from build123d import *

# Parameters (mm, degrees)
ESBO_O1_R                = 1
RESSALTO_EXTRUS_O1_DEPTH = 2.6
ESBO_O2_W                = 9.5
ESBO_O2_H                = 2.6
RESSALTO_EXTRUS_O2_DEPTH = 6
RESSALTO_EXTRUS_O2_TAPER = -20
RESSALTO_EXTRUS_O3_DEPTH = 5


with BuildPart() as part:
    # Esboço1 → Ressalto-extrusão1 (new body)
    with BuildSketch(Plane.XY):
        Polygon((-2.5, 31), (2.5, 31), (2.5, 19), (4.75, 19), (4.75, 0), (-4.75, 0), (-4.75, 19), (-2.5, 19), align=None)
        with Locations((0, 14)):
            Circle(ESBO_O1_R, mode=Mode.SUBTRACT)
    extrude(amount=RESSALTO_EXTRUS_O1_DEPTH)

    # Esboço2 → Ressalto-extrusão2 (add)
    with BuildSketch(Plane.XZ):
        with Locations((0, 1.3)):
            Rectangle(ESBO_O2_W, ESBO_O2_H)
    extrude(amount=-RESSALTO_EXTRUS_O2_DEPTH, taper=RESSALTO_EXTRUS_O2_TAPER)

    # Esboço3 → Ressalto-extrusão3 (add)
    with BuildSketch(Plane(origin=(2.5, 0, 0), x_dir=(0, 0, -1), z_dir=(1, 0, 0))):
        Polygon((-2.6, 31), (-3.6, 31), (-2.6, 25), align=None)
    extrude(amount=-RESSALTO_EXTRUS_O3_DEPTH)


solid = part.part
Geometry check sheet. Reference: the model listing, model coordinates, mm. A direction names the side the tool comes from. Give positions to 0.01 mm unless a question says otherwise; leave off trailing zeros. Order: outer loops, then holes, each group sorted by start corner. A loop starts at its lowest first (then second) coordinate and runs counter-clockwise, first axis right, second up. Notation, with made-up numbers: M -14.5,48 L 0.5,48 A26 ccw 0.5,73 Z; hole C 15,-23 d9. An arc over 180 degrees is marked long. Use a Markdown table: item, result.
Item 1: Depth check by flat-ended pin: P1, Ø7.5, axis at x = 2.5, y = 21, coming from the -Z side; P2, Ø1.6, axis at x = 0, y = 14, coming from the +Z side; P3, Ø3, axis at y = 14.5, z = 2, coming from the +X side; P4, Ø1.1, axis at y = 27.5, z = 2, coming from the +X side. Enter the tip coordinate at first touch or a pass-through.
Answers follow:
| item | result |
|---|---|
| P1 | stops at z = 0 |
| P2 | passes through |
| P3 | stops at x = 4.75 |
| P4 | stops at x = 2.5 |
Item 2: Section check A-A (y = 14). Record the cut outline in (x, z), and give its area (3 significant figures).
Answers follow:
| item | result |
|---|---|
| outline | M -4.75,0 L -1,0 L -1,2.6 L -4.75,2.6 Z; M 1,0 L 4.75,0 L 4.75,2.6 L 1,2.6 Z |
| area | 19.5 mm2 |
Item 3: Draft check along X on faces 1 (the cylindrical face through (0, 13, 1)), 2 (the flat face through (-4.75, 12, 1)), 3 (the flat face through (-4, 19, 1)). Enter one of: +X half, -X half, draft (parallel to the pull), parting line (faces both ways), or undercut.
Answers follow:
| item | result |
|---|---|
| face 1 | undercut |
| face 2 | -X half |
| face 3 | draft |
Item 4: Tool access check on faces 4 (the flat face through (0, 16, 0)), 5 (the flat face through (-2.5, 25, 1)), 6 (the flat face through (0, 31, 2)), 7 (the flat face through (0, 28, 3.1)), 8 (the flat face through (4.75, 13, 1)). Record the directions out of +Z, -Z, +X, -X, +Y, -Y that give a thin tool (end or side, any length) a straight path to the whole face; none if there is none.
Answers follow:
| item | result |
|---|---|
| face 4 | -Z, +X, -X, +Y |
| face 5 | +Z, -Z, -X, +Y |
| face 6 | +Z, -Z, +X, -X, +Y |
| face 7 | +Z, +X, -X |
| face 8 | +Z, -Z, +X, +Y |
Item 5: Material ranges on line 1 along Y through (x, z) = (0, 1.9); line 2 along Y through (x, z) = (-2.75, 1.5); line 3 along Z through (x, y) = (4, 15), recorded low to high.
Answers follow:
| item | result |
|---|---|
| line 1 | y = 0 to 13, 15 to 31 |
| line 2 | y = 0 to 19 |
| line 3 | z = 0 to 2.6 |
Item 6: Section check B-B (y = 20.5). Record the cut outline in (x, z), and give its area (3 significant figures).
Answers follow:
| item | result |
|---|---|
| outline | M -2.5,0 L 2.5,0 L 2.5,2.6 L -2.5,2.6 Z |
| area | 13.0 mm2 |
